from build123d import *

# Parameters (mm, degrees)
SKETCH1_W           = 6.35
SKETCH1_H           = 38.1
BOSS_EXTRUDE1_DEPTH = 50.8
SKETCH2_W           = 6.35
SKETCH2_H           = 12.7
BOSS_EXTRUDE2_DEPTH = 6.35
CUT_EXTRUDE1_DEPTH  = 55.624765446


with BuildPart() as part:
    # Sketch1 → Boss-Extrude1 (new body)
    with BuildSketch(Plane.XY):
        with Locations((-14.605, 0)):
            Rectangle(SKETCH1_W, SKETCH1_H)
    extrude(amount=BOSS_EXTRUDE1_DEPTH)

    # Sketch2 → Boss-Extrude2 (add)
    with BuildSketch(Plane(origin=(0, 0, 0), x_dir=(-1, 0, 0), z_dir=(0, 0, -1))):
        with Locations((14.605, -12.7)):
            Rectangle(SKETCH2_W, SKETCH2_H)
        with Locations((14.605, 12.7)):
            Rectangle(SKETCH2_W, SKETCH2_H)
    boss_extrude2 = extrude(amount=BOSS_EXTRUDE2_DEPTH)

    # Sketch3 → Cut-Extrude1 (cut, through all)
    with BuildSketch(Plane.ZY.offset(17.78)):
        Polygon((0, 2.1336), (0, -2.1336), (8.763, -2.1336), (8.763, -4.445), (11.938, -4.445), (11.938, -2.1336), (15.24, -2.1336), (15.24, 2.1336), (11.938, 2.1336), (11.938, 4.445), (8.763, 4.445), (8.763, 2.1336), align=None)
    cut_extrude1 = extrude(amount=-CUT_EXTRUDE1_DEPTH, mode=Mode.SUBTRACT)

    # Mirror1: Boss-Extrude2, Cut-Extrude1 across plane
    add(boss_extrude2.mirror(Plane.XY.offset(25.4)))
    add(cut_extrude1.mirror(Plane.XY.offset(25.4)), mode=Mode.SUBTRACT)


solid = part.part
Read the model definition and answer for the solid it produces. Units are mm, in the model's axes. A direction names the side the tool comes from. Give positions to 0.01 mm unless a question says otherwise; leave off trailing zeros. Write each loop counter-clockwise with the first axis right and the second up, starting at its lowest first coordinate (ties: lowest second). Pieces come first, ordered by that corner, then holes. Notation, with made-up numbers: (6, 9) - (33, 9) arc R18 cw to (33, 32) - close; hole circle Ø11 at (65.5, 1.25). An arc over 180 degrees is marked (long way). Return JSON: item names as keys, results as strings.
Q1. Given P1, Ø1.3, axis at x = -14.5, y = 0, coming from the +Z side; P2, Ø1.2, axis at x = -14, y = 3.5, coming from the +Z side; P3, Ø2.5, axis at x = -13.5, y = -3, coming from the -Z side, each flat-ended and moving along its own axis, determine where each tip first touches the part or whether it passes through.
Reply:
{"P1": "z = 35.56", "P2": "z = 50.8", "P3": "z = 0"}
Q2. A cutting plane is placed at C-C, the plane y = -5.5. Determine the outline of the cut face in (x, z).
Reply:
{"outline": "(-17.78, 0) - (-11.43, 0) - (-11.43, 50.8) - (-17.78, 50.8) - close"}
Q3. Consider line 1 along Z through (x, y) = (-15.5, 4); line 2 along Y through (x, z) = (-17.5, 38.5); line 3 along Z through (x, y) = (-13.75, 5.5). Determine where each line is inside the solid, lowest interval first. Write a range as [from, to].
Reply:
{"line 1": "[0, 8.76], [11.94, 38.86], [42.04, 50.8]", "line 2": "[-19.05, -2.13], [2.13, 19.05]", "line 3": "[0, 50.8]"}
Q4. A cutting plane is placed at A-A, the plane z = -1. Determine the outline of the cut face in (x, y).
Reply:
{"outline": "(-17.78, -19.05) - (-11.43, -19.05) - (-11.43, -6.35) - (-17.78, -6.35) - close; (-17.78, 6.35) - (-11.43, 6.35) - (-11.43, 19.05) - (-17.78, 19.05) - close"}
Q5. For faces 1 (the face through (-15, -2.134, 37)), 2 (the face through (-15, -6.35, -3)), 3 (the face through (-15, 4.445, 40)), determine the directions among +Z, -Z, +X, -X, +Y, -Y from which every point of the face is accessible in a straight line to the end or side of a thin tool.
Reply:
{"face 1": "+Z, +X, -X", "face 2": "-Z, +X, -X", "face 3": "+X, -X"}
Q6. A cutting plane is placed at B-B, the plane z = 6.5. Determine the outline of the cut face in (x, y).
Reply:
{"outline": "(-17.78, -19.05) - (-11.43, -19.05) - (-11.43, -2.13) - (-17.78, -2.13) - close; (-17.78, 2.13) - (-11.43, 2.13) - (-11.43, 19.05) - (-17.78, 19.05) - close"}
Q7. For a pull along Z with two mould halves and no side action, classify faces 4 (the face through (-15, -2.134, 14)), 5 (the face through (-15, -3, 38.862)), 6 (the face through (-15, -13, -6.35)) as released by +Z, released by -Z, zero draft, split by the parting line, or undercut.
Reply:
{"face 4": "zero draft", "face 5": "undercut", "face 6": "released by -Z"}
